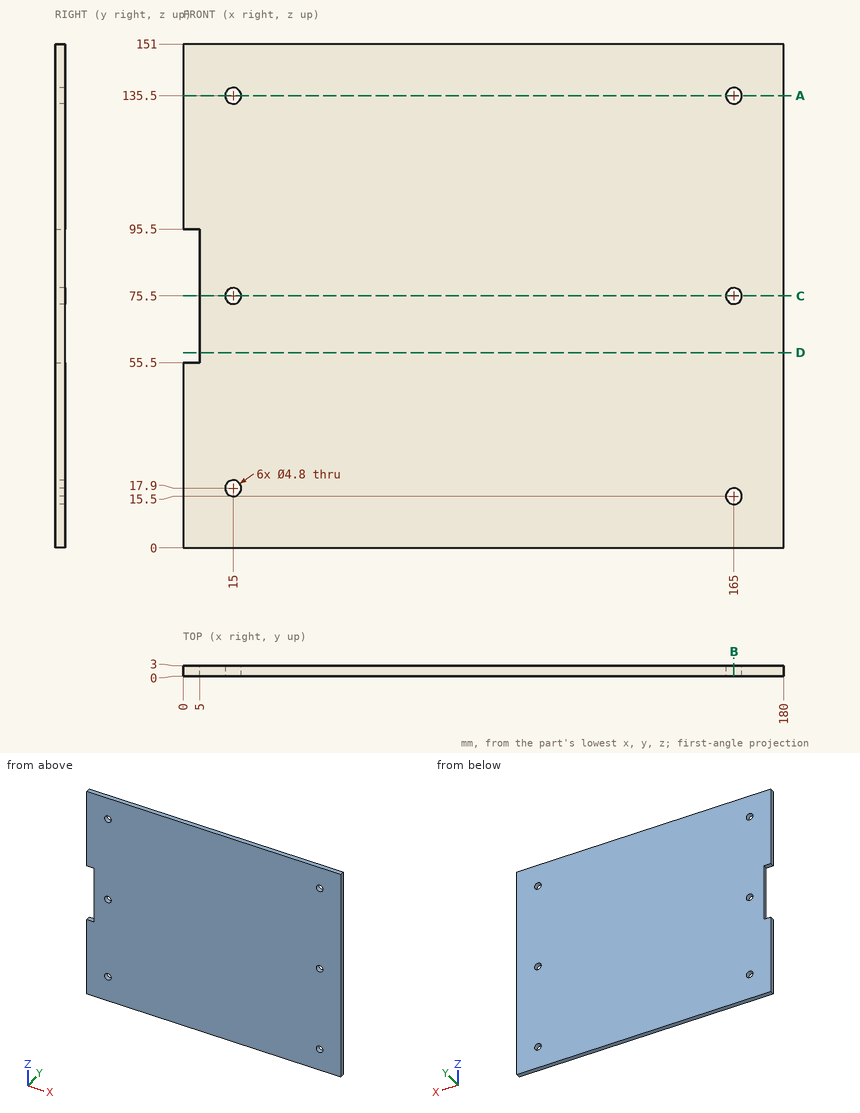
Check sheet for the drawn part. Datum: minimum x, y, z corner. Units: mm. Round coordinates to 2 decimals unless told otherwise and drop trailing zeros. Loops run counter-clockwise (first coordinate to the right, second up) from the corner with the lowest first, then second, coordinate; pieces in that order, holes last. Notation, with made-up numbers: M 82.25,66.25 L 138.25,66.25 A24 cw 138.25,101.25 Z; hole C 87.5,20 d5. An arc over 180 degrees is marked long. One line per question, with ' | ' between items. Start each with the question number.
Item 1: Section check C-C (z = 75.5). Record the boundary of the cut face in (x, y), and give its area (3 significant figures).
Item 2: Section check A-A (z = 135.5). Record the boundary of the cut face in (x, y), and give its area (3 significant figures).
Item 3: Section check B-B (x = 165). Record the boundary of the cut face in (y, z).
Item 4: Section check D-D (z = 58.5). Record the boundary of the cut face in (x, y).
Item 5: Scan lines: probe 1 along X at (y, z) = (2.05, 135.5); probe 2 along Z at (x, y) = (165, 2.25); probe 3 along Z at (x, y) = (15, 2). Record each from-to range of solid material in increasing order.
Item 6: Gauge pin test, flat ends, axial feed: pin 1 Ø7.5 at (x, z) = (165, 135.5) entering from +Y; pin 2 Ø1.5 at (y, z) = (1, 73.5) entering from -X. Record the tip position at first contact, or that the pin passes through.
Worked out:
1) outline: M 5,0 L 12.6,0 L 12.6,3 L 5,3 Z; M 17.4,0 L 162.6,0 L 162.6,3 L 17.4,3 Z; M 167.4,0 L 180,0 L 180,3 L 167.4,3 Z | area: 496 mm^2
2) outline: M 0,0 L 12.6,0 L 12.6,3 L 0,3 Z; M 17.4,0 L 162.6,0 L 162.6,3 L 17.4,3 Z; M 167.4,0 L 180,0 L 180,3 L 167.4,3 Z | area: 511 mm^2
3) outline: M 0,0 L 3,0 L 3,13.1 L 0,13.1 Z; M 0,17.9 L 3,17.9 L 3,73.1 L 0,73.1 Z; M 0,77.9 L 3,77.9 L 3,133.1 L 0,133.1 Z; M 0,137.9 L 3,137.9 L 3,151 L 0,151 Z
4) outline: M 5,0 L 180,0 L 180,3 L 5,3 Z
5) probe 1: 0 to 12.6, 17.4 to 162.6, 167.4 to 180 | probe 2: 0 to 13.1, 17.9 to 73.1, 77.9 to 133.1, 137.9 to 151 | probe 3: 0 to 15.5, 20.3 to 73.1, 77.9 to 133.1, 137.9 to 151
6) pin 1: y = 3 | pin 2: x = 5
